Geometry: final body of the model. Coordinates: model frame, mm. Face numbers are marked on the shaded views. A direction names the side the tool comes from. Coordinates: 2 decimals unless noted, no trailing zeros. Write each loop counter-clockwise with the first axis right and the second up, starting at its lowest first coordinate (ties: lowest second). Pieces come first, ordered by that corner, then holes.
from build123d import *

# Parameters (mm, degrees)
SKETCH1_W                = 15
SKETCH1_H                = 15
SKETCH1_R                = 2.5
BOSS_EXTRUDE1_DEPTH      = 3
CHAMFER1_SIZE            = 3
SKETCH1_6_R              = 2.5
BOSS_EXTRUDE3_DEPTH      = 0.5
SKETCH18_W               = 9
SKETCH18_H               = 9
CHAMFER4_SIZE            = 4
CHAMFER5_SIZE            = 3
SKETCH19_OUTSIDE_W       = 25.408
SKETCH19_OUTSIDE_H       = 24.908
SKETCH19_OUTSIDE_R       = 2.5
CUT_EXTRUDE2_DEPTH       = 5
F_3_0_3_DIAMETER_HOLE1_D = 3


with BuildPart() as part:
    # Sketch1 → Boss-Extrude1 (new body)
    with BuildSketch(Plane(origin=(0, 0, 0), x_dir=(1, 0, 0), z_dir=(0, 1, 0))):
        Rectangle(SKETCH1_W, SKETCH1_H)
        with Locations(Location((0, 0, 0), (0, 0, 270))):
            Circle(SKETCH1_R, mode=Mode.SUBTRACT)
    extrude(amount=BOSS_EXTRUDE1_DEPTH)

    # Chamfer1
    chamfer1_edges = [part.edges().sort_by_distance(p)[0] for p in [
        (7.5, 1.5, 7.5),
        (-7.5, 1.5, 7.5),
        (-7.5, 1.5, -7.5),
        (7.5, 1.5, -7.5),
    ]]
    chamfer(chamfer1_edges, length=CHAMFER1_SIZE)

    # Sketch1<6> → Boss-Extrude3 (add)
    with BuildSketch(Plane(origin=(0, 0, 0), x_dir=(1, 0, 0), z_dir=(0, 1, 0))):
        with Locations(Location((0, 0, 0), (0, 0, 270))):
            Circle(SKETCH1_6_R)
    extrude(amount=BOSS_EXTRUDE3_DEPTH)

    # Sweep3: sweep along a path in Sketch2
    with BuildLine(Plane(origin=(0, 0, 0), x_dir=(0, 0, -1), z_dir=(1, 0, 0))) as sweep3_path:
        Line((0, 0), (0, -7))
        Line((0, -7), (29, -7))
    # Sketch18 → Sweep3 (sweep)
    with BuildSketch(Plane.XZ):
        Rectangle(SKETCH18_W, SKETCH18_H)
    sweep(path=sweep3_path.line, transition=Transition.RIGHT)

    # Chamfer4
    # the kernel refuses this chamfer: 4 mm, written as the material it adds along each edge
    with BuildSketch(Plane(origin=(-14.786731952, 0, -4.5), x_dir=(0, 0, -1), z_dir=(1, 0, 0))) as chamfer4_piece_1_section:
        Polygon((CHAMFER4_SIZE, 0), (0, -CHAMFER4_SIZE), (0, 0), align=None)
    chamfer4_piece_1 = extrude(amount=29.573463904, mode=Mode.PRIVATE)
    chamfer4_piece_1 = split(chamfer4_piece_1, bisect_by=Plane(origin=(-14.786731952, 0, -7.5), z_dir=(0, 0, 1)), keep=Keep.TOP, mode=Mode.PRIVATE)
    chamfer4_piece_1 = split(chamfer4_piece_1, bisect_by=Plane(origin=(-11.143365976, 0, -0.856634024), z_dir=(0.7071067811865476, 0, 0.7071067811865476)), keep=Keep.TOP, mode=Mode.PRIVATE)
    chamfer4_piece_1 = split(chamfer4_piece_1, bisect_by=Plane(origin=(-3.643365976, 0, -15.643365976), z_dir=(-0.7071067811865476, 0, 0.7071067811865476)), keep=Keep.TOP, mode=Mode.PRIVATE)
    chamfer4_piece_1 = split(chamfer4_piece_1, bisect_by=Plane(origin=(-11.643365976, 3.143365976, -4.5), z_dir=(0.7071067811865476, 0.7071067811865475, 0)), keep=Keep.TOP, mode=Mode.PRIVATE)
    chamfer4_piece_1 = split(chamfer4_piece_1, bisect_by=Plane(origin=(-3.143365976, -11.643365976, -4.5), z_dir=(-0.7071067811865476, 0.7071067811865475, 0)), keep=Keep.TOP, mode=Mode.PRIVATE)
    add(chamfer4_piece_1)
    with BuildSketch(Plane(origin=(4.5, 0, -14.786731952), x_dir=(1, 0, 0), z_dir=(0, 0, 1))) as chamfer4_piece_2_section:
        Polygon((CHAMFER4_SIZE, 0), (0, -CHAMFER4_SIZE), (0, 0), align=None)
    chamfer4_piece_2 = extrude(amount=29.573463904, mode=Mode.PRIVATE)
    chamfer4_piece_2 = split(chamfer4_piece_2, bisect_by=Plane(origin=(0.856634024, 0, -11.143365976), z_dir=(-0.7071067811865476, 0, 0.7071067811865476)), keep=Keep.TOP, mode=Mode.PRIVATE)
    chamfer4_piece_2 = split(chamfer4_piece_2, bisect_by=Plane(origin=(7.5, 0, -14.786731952), z_dir=(-1, 0, 0)), keep=Keep.TOP, mode=Mode.PRIVATE)
    chamfer4_piece_2 = split(chamfer4_piece_2, bisect_by=Plane(origin=(15.643365976, 0, -3.643365976), z_dir=(-0.7071067811865476, 0, -0.7071067811865476)), keep=Keep.TOP, mode=Mode.PRIVATE)
    chamfer4_piece_2 = split(chamfer4_piece_2, bisect_by=Plane(origin=(4.5, 3.143365976, -11.643365976), z_dir=(0, 0.7071067811865475, 0.7071067811865476)), keep=Keep.TOP, mode=Mode.PRIVATE)
    chamfer4_piece_2 = split(chamfer4_piece_2, bisect_by=Plane(origin=(4.5, -11.643365976, -3.143365976), z_dir=(0, 0.7071067811865477, -0.7071067811865475)), keep=Keep.TOP, mode=Mode.PRIVATE)
    add(chamfer4_piece_2)
    with BuildSketch(Plane(origin=(14.786731952, 0, 4.5), x_dir=(0, 0, 1), z_dir=(-1, 0, 0))) as chamfer4_piece_3_section:
        Polygon((CHAMFER4_SIZE, 0), (0, -CHAMFER4_SIZE), (0, 0), align=None)
    chamfer4_piece_3 = extrude(amount=29.573463904, mode=Mode.PRIVATE)
    chamfer4_piece_3 = split(chamfer4_piece_3, bisect_by=Plane(origin=(3.643365976, 0, 15.643365976), z_dir=(0.7071067811865476, 0, -0.7071067811865476)), keep=Keep.TOP, mode=Mode.PRIVATE)
    chamfer4_piece_3 = split(chamfer4_piece_3, bisect_by=Plane(origin=(11.143365976, 0, 0.856634024), z_dir=(-0.7071067811865476, 0, -0.7071067811865476)), keep=Keep.TOP, mode=Mode.PRIVATE)
    chamfer4_piece_3 = split(chamfer4_piece_3, bisect_by=Plane(origin=(14.786731952, 0, 7.5), z_dir=(0, 0, -1)), keep=Keep.TOP, mode=Mode.PRIVATE)
    chamfer4_piece_3 = split(chamfer4_piece_3, bisect_by=Plane(origin=(3.143365976, -11.643365976, 4.5), z_dir=(0.7071067811865476, 0.7071067811865475, 0)), keep=Keep.TOP, mode=Mode.PRIVATE)
    chamfer4_piece_3 = split(chamfer4_piece_3, bisect_by=Plane(origin=(11.643365976, 3.143365976, 4.5), z_dir=(-0.7071067811865476, 0.7071067811865475, 0)), keep=Keep.TOP, mode=Mode.PRIVATE)
    add(chamfer4_piece_3)
    with BuildSketch(Plane(origin=(-4.5, 0, 14.786731952), x_dir=(-1, 0, 0), z_dir=(0, 0, -1))) as chamfer4_piece_4_section:
        Polygon((CHAMFER4_SIZE, 0), (0, -CHAMFER4_SIZE), (0, 0), align=None)
    chamfer4_piece_4 = extrude(amount=29.573463904, mode=Mode.PRIVATE)
    chamfer4_piece_4 = split(chamfer4_piece_4, bisect_by=Plane(origin=(-15.643365976, 0, 3.643365976), z_dir=(0.7071067811865476, 0, 0.7071067811865476)), keep=Keep.TOP, mode=Mode.PRIVATE)
    chamfer4_piece_4 = split(chamfer4_piece_4, bisect_by=Plane(origin=(-7.5, 0, 14.786731952), z_dir=(1, 0, 0)), keep=Keep.TOP, mode=Mode.PRIVATE)
    chamfer4_piece_4 = split(chamfer4_piece_4, bisect_by=Plane(origin=(-0.856634024, 0, 11.143365976), z_dir=(0.7071067811865476, 0, -0.7071067811865476)), keep=Keep.TOP, mode=Mode.PRIVATE)
    chamfer4_piece_4 = split(chamfer4_piece_4, bisect_by=Plane(origin=(-4.5, -11.643365976, 3.143365976), z_dir=(0, 0.7071067811865475, 0.7071067811865476)), keep=Keep.TOP, mode=Mode.PRIVATE)
    chamfer4_piece_4 = split(chamfer4_piece_4, bisect_by=Plane(origin=(-4.5, 3.143365976, 11.643365976), z_dir=(0, 0.7071067811865477, -0.7071067811865475)), keep=Keep.TOP, mode=Mode.PRIVATE)
    add(chamfer4_piece_4)

    # Chamfer5
    # the kernel refuses this chamfer: 3 mm, written as the material it takes off along each edge
    with BuildSketch(Plane(origin=(4.5, -11.5, 12.215048964), x_dir=(-1, 0, 0), z_dir=(0, 0, -1))) as chamfer5_piece_1:
        Polygon((CHAMFER5_SIZE, 0), (0, CHAMFER5_SIZE), (0, 0), align=None)
    extrude(amount=48.930097928, mode=Mode.SUBTRACT)
    with BuildSketch(Plane(origin=(-4.5, -11.5, 12.215048964), x_dir=(1, 0, 0), z_dir=(0, 0, -1))) as chamfer5_piece_2:
        Polygon((CHAMFER5_SIZE, 0), (0, -CHAMFER5_SIZE), (0, 0), align=None)
    extrude(amount=48.930097928, mode=Mode.SUBTRACT)
    with BuildSketch(Plane(origin=(4.5, -2.5, 1.715048964), x_dir=(-1, 0, 0), z_dir=(0, 0, -1))) as chamfer5_piece_3_section:
        Polygon((CHAMFER5_SIZE, 0), (0, -CHAMFER5_SIZE), (0, 0), align=None)
    chamfer5_piece_3 = extrude(amount=38.430097928, mode=Mode.PRIVATE)
    chamfer5_piece_3 = split(chamfer5_piece_3, bisect_by=Plane(origin=(4.5, -6.357524482, -2.142475518), z_dir=(0, -0.7071067811865476, -0.7071067811865476)), keep=Keep.TOP, mode=Mode.PRIVATE)
    add(chamfer5_piece_3, mode=Mode.SUBTRACT)
    with BuildSketch(Plane(origin=(-4.5, -2.5, 1.715048964), x_dir=(1, 0, 0), z_dir=(0, 0, -1))) as chamfer5_piece_4_section:
        Polygon((CHAMFER5_SIZE, 0), (0, CHAMFER5_SIZE), (0, 0), align=None)
    chamfer5_piece_4 = extrude(amount=38.430097928, mode=Mode.PRIVATE)
    chamfer5_piece_4 = split(chamfer5_piece_4, bisect_by=Plane(origin=(-4.5, -6.357524482, -2.142475518), z_dir=(0, -0.7071067811865476, -0.7071067811865476)), keep=Keep.TOP, mode=Mode.PRIVATE)
    add(chamfer5_piece_4, mode=Mode.SUBTRACT)
    with BuildSketch(Plane(origin=(4.5, 3.715048964, 4.5), x_dir=(-1, 0, 0), z_dir=(0, -1, 0))) as chamfer5_piece_5_section:
        Polygon((CHAMFER5_SIZE, 0), (0, CHAMFER5_SIZE), (0, 0), align=None)
    chamfer5_piece_5 = extrude(amount=22.930097928, mode=Mode.PRIVATE)
    chamfer5_piece_5 = split(chamfer5_piece_5, bisect_by=Plane(origin=(8.357524482, -0.142475518, 4.5), z_dir=(0.7071067811865476, -0.7071067811865476, 0)), keep=Keep.TOP, mode=Mode.PRIVATE)
    add(chamfer5_piece_5, mode=Mode.SUBTRACT)
    with BuildSketch(Plane(origin=(4.5, 3.715048964, 4.5), x_dir=(-1, 0, 0), z_dir=(0, -1, 0))) as chamfer5_piece_6_section:
        Polygon((CHAMFER5_SIZE, 0), (0, CHAMFER5_SIZE), (0, 0), align=None)
    chamfer5_piece_6 = extrude(amount=22.930097928, mode=Mode.PRIVATE)
    chamfer5_piece_6 = split(chamfer5_piece_6, bisect_by=Plane(origin=(4.5, -0.142475518, 8.357524482), z_dir=(0, -0.7071067811865476, 0.7071067811865476)), keep=Keep.TOP, mode=Mode.PRIVATE)
    add(chamfer5_piece_6, mode=Mode.SUBTRACT)
    with BuildSketch(Plane(origin=(-4.5, 3.715048964, 4.5), x_dir=(1, 0, 0), z_dir=(0, -1, 0))) as chamfer5_piece_7_section:
        Polygon((CHAMFER5_SIZE, 0), (0, -CHAMFER5_SIZE), (0, 0), align=None)
    chamfer5_piece_7 = extrude(amount=22.930097928, mode=Mode.PRIVATE)
    chamfer5_piece_7 = split(chamfer5_piece_7, bisect_by=Plane(origin=(-8.357524482, -0.142475518, 4.5), z_dir=(-0.7071067811865476, -0.7071067811865476, 0)), keep=Keep.TOP, mode=Mode.PRIVATE)
    add(chamfer5_piece_7, mode=Mode.SUBTRACT)
    with BuildSketch(Plane(origin=(-4.5, 3.715048964, 4.5), x_dir=(1, 0, 0), z_dir=(0, -1, 0))) as chamfer5_piece_8_section:
        Polygon((CHAMFER5_SIZE, 0), (0, -CHAMFER5_SIZE), (0, 0), align=None)
    chamfer5_piece_8 = extrude(amount=22.930097928, mode=Mode.PRIVATE)
    chamfer5_piece_8 = split(chamfer5_piece_8, bisect_by=Plane(origin=(-4.5, -0.142475518, 8.357524482), z_dir=(0, -0.7071067811865476, 0.7071067811865476)), keep=Keep.TOP, mode=Mode.PRIVATE)
    add(chamfer5_piece_8, mode=Mode.SUBTRACT)

    # Sketch19 outside → Cut-Extrude2 (cut)
    with BuildSketch(Plane(origin=(0, 0, -29), x_dir=(-1, 0, 0), z_dir=(0, 0, -1))):
        with Locations((0, -4.25)):
            Rectangle(SKETCH19_OUTSIDE_W, SKETCH19_OUTSIDE_H)
        with Locations(Location((0, -7, 0), (0, 0, 90))):
            Circle(SKETCH19_OUTSIDE_R, mode=Mode.SUBTRACT)
    extrude(amount=-CUT_EXTRUDE2_DEPTH, mode=Mode.SUBTRACT)

    # Ø3.0 (3) Diameter Hole1 (through all)
    with Locations(Plane(origin=(0, 3, 0), x_dir=(1, 0, 0), z_dir=(0, 1, 0))):
        with Locations((0, 0)):
            Hole(F_3_0_3_DIAMETER_HOLE1_D / 2)


solid = part.part
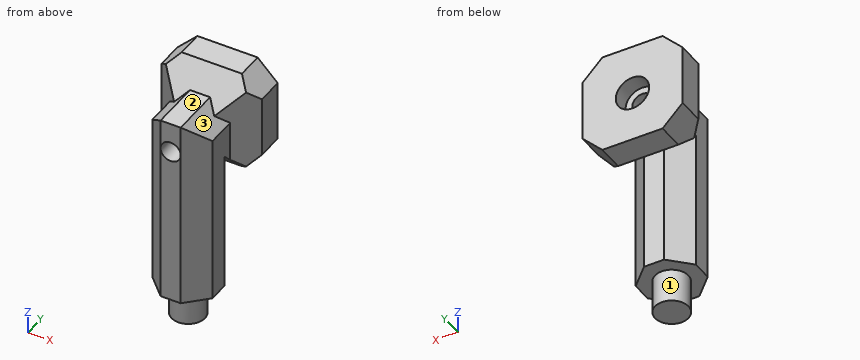
Item 1: Section D-D, the plane x = -5.5. Output: boundary loops of the cut face in (y, z).
Derived:
outline: (-3, -5.5) - (-2, -6.5) - (3, -6.5) - (3, 6.5) - (-2, 6.5) - (-3, 5.5) - close
Item 2: Section C-C, the plane z = -3.5. Output: boundary loops of the cut face in (x, y).
Derived:
outline: (-7.5, -1) - (-4.5, -4) - (-4.5, -5) - (-4, -5) - (-4.5, -5.5) - (-4.5, -8.5) - (-1.5, -11.5) - (1.5, -11.5) - (4.5, -8.5) - (4.5, -5.5) - (4, -5) - (4.5, -5) - (4.5, -4) - (7.5, -1) - (7.5, 3) - (-7.5, 3) - close
Item 3: Pin query (flat end, axial travel): pin 1 (1.5 mm diameter, centred on x = -3.5, z = -23.5, fed in from +Y); pin 2 (4 mm diameter, centred on x = 0, y = -1.5, fed in from -Z); pin 3 (1 mm diameter, centred on x = 3, z = -23.5, fed in from +Y). Return the tip coordinate at first contact, or that it passes through.
Derived:
pin 1: stops at y = -3.75
pin 2: stops at z = -24
pin 3: stops at y = -3.5
Item 4: Material intervals for probe 1 along X at (y, z) = (1.2, 0); probe 2 along Z at (x, y) = (0, -4); probe 3 along Z at (x, y) = (0, -7.5), sorted ascending.
Derived:
probe 1: x = -7.5 to -2.5, 2.5 to 7.5
probe 2: z = -24 to -1.5, 1.5 to 4.5
probe 3: z = -29 to -1.5, 1.5 to 4.5
Item 5: Section A-A, the plane x = 0. Output: boundary loops of the cut face in (y, z).
Derived:
outline: (-11.5, -24) - (-9.5, -24) - (-9.5, -29) - (-4.5, -29) - (-4.5, -24) - (-2.5, -24) - (-2.5, -6) - (-1, -7.5) - (3, -7.5) - (3, -2.5) - (0.5, -2.5) - (0.5, -1.5) - (-11.5, -1.5) - close; (-11.5, 1.5) - (0.5, 1.5) - (0.5, 2.5) - (3, 2.5) - (3, 7.5) - (-1, 7.5) - (-4, 4.5) - (-11.5, 4.5) - close
Item 6: Set-up query: the marked faces 1, 2 and 3. Return all of +Z, -Z, +X, -X, +Y, -Y with unobstructed straight access to the full face (end or side cutting, diameter ignored); none if empty.
Derived:
face 1: -Z
face 2: +Z, +X, -X, -Y
face 3: +Z, +X, -Y
Item 7: Section B-B, the plane y = 1. Output: boundary loops of the cut face in (x, z).
Derived:
outline: (-7.5, -4.5) - (-4.5, -7.5) - (4.5, -7.5) - (7.5, -4.5) - (7.5, 4.5) - (4.5, 7.5) - (-4.5, 7.5) - (-7.5, 4.5) - close; hole circle Ø5 at (0, 0)
